from build123d import *

# Parameters (mm, degrees)
EXTRUDE_1_DEPTH = 4


with BuildPart() as part:
    # Эскиз1 → Бобышка-Вытянуть1 (new body)
    with BuildSketch(Plane.XY):
        Polygon((0, 0), (48, 0), (39.231886792, 57), (4.301886792, 57), align=None)
        with BuildLine():
            Line((4.414773297, 5.495746181), (7.887113496, 51.504253819))
            ThreePointArc((7.887113496, 51.504253819), (6.980031804, 54.099847661), (9.5, 53))
            Line((9.5, 53), (31.5, 53))
            ThreePointArc((31.5, 53), (33.94432859, 54.165437048), (33.310991351, 51.532592633))
            Line((33.310991351, 51.532592633), (43.073702459, 5.467407367))
            ThreePointArc((43.073702459, 5.467407367), (44.550130858, 3.05567141), (41.88469381, 4))
            Line((41.88469381, 4), (5.801886792, 4))
            ThreePointArc((5.801886792, 4), (3.202039131, 2.980031804), (4.414773297, 5.495746181))
        make_face(mode=Mode.SUBTRACT)
    extrude(amount=EXTRUDE_1_DEPTH)


solid = part.part
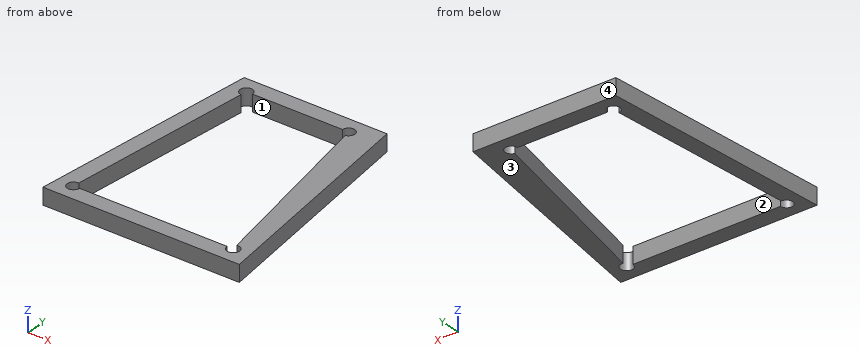
The model under review builds one solid part; all positions refer to its coordinate system, in mm. Face numbers are marked on the shaded views. Coordinates: 2 decimals unless noted, no trailing zeros. Loops run counter-clockwise (first coordinate to the right, second up) from the corner with the lowest first, then second, coordinate; pieces in that order, holes last. Notation, with made-up numbers: M 4,3 L 19,3 A12 cw 19,12 Z; hole C 50,-9.5 d4. An arc over 180 degrees is marked long. Put each result on its own line as item: value. Start each with the question number.
Q1. Add section C-C (z = 1). Write out the cut boundary in (x, y), and give its area (3 significant figures).
Q2. Add section A-A (x = 27). Write out the cut boundary in (y, z), and give its area (3 significant figures).
Q3. Wall thickness on line 1 (Y direction, x = 15.5, z = 2.75); line 2 (Y direction, x = 8, z = 2.3); line 3 (X direction, y = 6, z = 1.2): over which ranges is each line inside the solid? List them lowest first.
Q4. The part is to be moulded in two halves that separate along Y. For the marked faces 1, 2, 3 and 4, say which applies: +Y half, -Y half, draft (parallel to the pull), parting line (faces both ways), or undercut.
Q5. Add section B-B (y = 21). Write out the cut boundary in (x, z), and give its area (3 significant figures).
Answers:
1. outline: M 0,0 L 48,0 L 39.23,57 L 4.3,57 Z; hole M 4.41,5.5 A1.5 ccw long 5.8,4 L 41.88,4 A1.5 ccw long 43.07,5.47 L 33.31,51.53 A1.5 ccw long 31.5,53 L 9.5,53 A1.5 ccw long 7.89,51.5 Z
1. area: 772 mm^2
2. outline: M 0,0 L 4,0 L 4,4 L 0,4 Z; M 53,0 L 57,0 L 57,4 L 53,4 Z
2. area: 32.0 mm^2
3. line 1: y = 0 to 4, 53 to 57
3. line 2: y = 0 to 4, 54.5 to 57
3. line 3: x = 0.45 to 4.45, 42.96 to 47.08
4. face 1: undercut
4. face 2: undercut
4. face 3: draft
4. face 4: +Y half
5. outline: M 1.58,0 L 5.58,0 L 5.58,4 L 1.58,4 Z; M 39.78,0 L 44.77,0 L 44.77,4 L 39.78,4 Z
5. area: 36.0 mm^2
